Source: CAD feature listing. Evaluate the final solid. Frame: model axes, mm. A direction names the side the tool comes from. Give positions to 0.01 mm unless a question says otherwise; leave off trailing zeros. Loops run counter-clockwise (first coordinate to the right, second up) from the corner with the lowest first, then second, coordinate; pieces in that order, holes last. Notation, with made-up numbers: (-10.5, 70.25) -> (18.5, 70.25) arc R20 ccw to (18.5, 108.25) -> close; hole circle Ø1 at (61, 79). An arc over 180 degrees is marked (long way). Return JSON: item names as keys, results as strings. Group by question number.
(1) Ray query, line 1 (X direction, y = -388, z = 174.5); line 2 (Z direction, x = -580.5, y = 101.5). Return the intervals inside material, ascending. Write a range as from..to.
(2) Access query for faces 4 (the face through (1219.2, -6, -3)), 5 (the face through (-711.2, -6, -166)), 6 (the face through (508, -6, 165)). Directions: +Z, -Z, +X, -X, +Y, -Y. A direction counts if a zero-diameter tool reaches every point of the face in a straight line with its end or side. Return the directions, or none.
(3) Cut plane B-B on y = 113.5. Return loops of the section in (x, z).
(4) Draft query along X for faces 1 (the face through (-962, -6, 203.2)), 2 (the face through (-611, -6, -127)), 3 (the face through (-1219.2, -6, 3)). Return one class per face: released by +X, released by -X, zero draft, split by the parting line, or undercut.
(5) Pin query (flat end, axial travel): pin 1 (3 mm diameter, centred on x = 597.5, y = -327, fed in from -Z). Return the tip coordinate at first contact, or that it passes through.
(6) Cut plane A-A on z = -156. Return loops of the section in (x, y), then the cut area to 3 significant figures.
```python
from build123d import *

# Parameters (mm, degrees)
F1_DEPTH = 457.2


with BuildPart() as f1:
    # F0 (on Front) → F1 (new body, symmetric)
    with BuildSketch(Plane.XZ):
        Polygon((-711.2, 203.2), (-1219.2, 203.2), (-1219.2, -203.2), (-711.2, -203.2), (-711.2, -127), (-508, -127), (-508, -203.2), (508, -203.2), (508, -127), (711.2, -127), (711.2, -203.2), (1219.2, -203.2), (1219.2, 203.2), (711.2, 203.2), (711.2, 127), (508, 127), (508, 203.2), (-508, 203.2), (-508, 127), (-711.2, 127), align=None)
    extrude(amount=F1_DEPTH, both=True)


solid = f1.part
```
Answers:
{
 "1": {"line 1": "-1219.2..-711.2, -508..508, 711.2..1219.2", "line 2": "-127..127"},
 "2": {"face 4": "+Z, -Z, +X, +Y, -Y", "face 5": "-Z, +Y, -Y", "face 6": "+Z, +Y, -Y"},
 "3": {"outline": "(-1219.2, -203.2) -> (-711.2, -203.2) -> (-711.2, -127) -> (-508, -127) -> (-508, -203.2) -> (508, -203.2) -> (508, -127) -> (711.2, -127) -> (711.2, -203.2) -> (1219.2, -203.2) -> (1219.2, 203.2) -> (711.2, 203.2) -> (711.2, 127) -> (508, 127) -> (508, 203.2) -> (-508, 203.2) -> (-508, 127) -> (-711.2, 127) -> (-711.2, 203.2) -> (-1219.2, 203.2) -> close"},
 "4": {"face 1": "zero draft", "face 2": "undercut", "face 3": "released by -X"},
 "5": {"pin 1": "z = -127"},
 "6": {"outline": "(-1219.2, -457.2) -> (-711.2, -457.2) -> (-711.2, 457.2) -> (-1219.2, 457.2) -> close; (-508, -457.2) -> (508, -457.2) -> (508, 457.2) -> (-508, 457.2) -> close; (711.2, -457.2) -> (1219.2, -457.2) -> (1219.2, 457.2) -> (711.2, 457.2) -> close", "area": "1,860,000 mm²"}
}
